Autodesk Inventor part; units mm, degrees
ref_plane "YZ Plane" through (0, 0, 0) normal (1, 0, 0) x (0, 1, 0)
ref_plane "XZ Plane" through (0, 0, 0) normal (0, 1, 0) x (-1, 0, 0)
ref_plane "XY Plane" through (0, 0, 0) normal (0, 0, 1) x (1, 0, 0)
sketch "Sketch1" plane through (0, 0, 0) normal (0, 1, 0) x (-1, 0, 0)
  circle A0 centre (275.1702, 127.184) radius 4.5
  circle A1 centre (341.1702, 61.184) radius 4.5
  circle A2 centre (341.1702, 193.184) radius 4.5
  circle A3 centre (407.1702, 127.184) radius 4.5
  line L0 (404.6478, 74.313) -> (450.2561, 28.7046)
  arc A4 (450.2561, 28.7046) -> (457.1702, 51.184) centre (417.1702, 51.184) ccw
  line L1 (457.1702, 51.184) -> (457.1702, 311.184)
  line L2 (457.1702, 311.184) -> (122.1702, 311.184)
  line L3 (122.1702, 311.184) -> (122.1702, 11.184)
  line L4 (122.1702, 11.184) -> (417.1702, 11.184)
  arc A5 (417.1702, 11.184) -> (439.6495, 18.098) centre (417.1702, 51.184) ccw
  line L5 (439.6495, 18.098) -> (394.0412, 63.7064)
  arc A6 (404.6478, 74.313) -> (394.0412, 63.7064) centre (399.3445, 69.0097) ccw
  circle A7 centre (438.3202, 72.034) radius 11.75
  circle A8 centre (396.3202, 30.034) radius 11.75
  circle A9 centre (356.7202, 30.034) radius 7.85
  circle A10 centre (438.3202, 111.634) radius 7.85
  circle A11 centre (141.0202, 292.334) radius 7.85
  circle A12 centre (141.0202, 30.034) radius 7.85
  circle A13 centre (438.3202, 292.334) radius 7.85
  line L6 (122.1702, 11.184) -> (-212.8298, 11.184)
  line L7 (-212.8298, 11.184) -> (-212.8298, 311.184)
  line L8 (-212.8298, 311.184) -> (122.1702, 311.184)
  line L9 (122.1702, 311.184) -> (122.1702, 11.184)
  point P0 (0, 0)
  point P1 (-193.9798, 72.034)
  point P2 (-151.9798, 30.034)
  point P3 (-112.3798, 30.034)
  point P4 (-193.9798, 111.634)
  point P5 (103.3202, 292.334)
  point P6 (103.3202, 30.034)
  point P7 (-193.9798, 292.334)
  point P8 (103.3202, 292.334)
  point P9 (103.3202, 30.034)
  point P10 (-112.3798, 30.034)
  point P11 (-151.9798, 30.034)
  point P12 (-193.9798, 72.034)
  point P13 (-193.9798, 111.634)
  point P14 (-193.9798, 292.334)
  dimension "d0" = 335
  dimension "d1" = 300
  dimension "d2" = 0
  dimension "d3" = 0
extrude "Extrusion1" add sketch "Sketch1" against normal blind 10.5 contours L3 L6 L7 L8
hole "Hole2" at (-103.3202, 0, 292.334) at (-103.3202, 0, 30.034) at (112.3798, 0, 30.034) at (193.9798, 0, 111.634) at (193.9798, 0, 292.334) direction (0, -1, 0) diameter 8 end through all countersink diameter 15.7 countersink angle 90
hole "Hole3" at (151.9798, 0, 30.034) at (193.9798, 0, 72.034) direction (0, -1, 0) diameter 12 end through all countersink diameter 23.5 countersink angle 90
fillet "Fillet1" radius 40 1 edges at (212.8298, -5.25, 11.184)
properties part number "Right top plate"
Here's how the part is built. I have some questions about the finished solid (model axes, mm). Give positions to 0.01 mm unless a question says otherwise; leave off trailing zeros. Put each result on its own line as item: value. Start each with the question number.
Item 1: I need wall thicknesses on L1, parallel to Z at x = -103, y = -6; L2, parallel to Z at x = -100, y = -6.25; L3, parallel to X at y = -3.25, z = 34. Which ranges of each line are inside material? Lowest first, please. Write a range as from..to.
Item 2: Will these pins go through, and if not, where does the flat tip stop? pin 1 (19 mm diameter, centred on x = 151.98, z = 30.03, fed in from +Y); pin 2 (10.5 mm diameter, centred on x = -103.32, z = 292.33, fed in from +Y).
Item 3: Thinking about a two-plate mould opening in X: for faces 1 (the flat face through (48, -5, 311.184)), 2 (the conical face through (108.62, -3.61, 31.99)), 3 (the cylindrical face through (200.8, -5.32, 22.59)), which applies, +X half, -X half, draft (parallel to the pull), parting line (faces both ways), or undercut?
Item 4: If we section it at A-A, the plane z = 292: Count the separate pieces of the cut face and the enclosed holes in it, then the cut area to 3 significant figures.
Values:
1. L1: 11.18..26.05, 34.02..288.35, 296.32..311.18
1. L2: 11.18..27.8, 32.26..290.1, 294.56..311.18
1. L3: -122.17..-105.65, -100.99..110.05, 114.71..144.46, 159.5..208.95
2. pin 1: y = -2.25
2. pin 2: y = -2.6
3. face 1: draft
3. face 2: undercut
3. face 3: +X half
4. separate pieces: 3
4. enclosed holes: 0
4. area: 3,320 mm²
